```python
from build123d import *

# Parameters (mm, degrees)
PROFILE_R   = 4.7625
PROFILE_R_2 = 3.8735


with BuildPart() as part:
    # Tube: sweep along a curve in space
    with BuildLine() as tube_path:
        Line((-2198.887960479, -22.400788354, -83.600880265), (-2179.087960479, -22.400788354, -83.600880265))
        Line((-2179.087960479, -22.400788354, -83.600880265), (-2172.876303396, -22.612445436, -84.390795251))
        Line((-2172.876303396, -22.612445436, -84.390795251), (-2167.087960479, -23.232992603, -86.706708807))
        Line((-2167.087960479, -23.232992603, -86.706708807), (-2162.11739773, -24.220140591, -90.390795251))
        Line((-2162.11739773, -24.220140591, -90.390795251), (-2158.303350788, -25.506616895, -95.191990181))
        Line((-2158.303350788, -25.506616895, -95.191990181), (-2155.905740648, -27.004750281, -100.783100096))
        Line((-2155.905740648, -27.004750281, -100.783100096), (-2155.087960479, -28.612445436, -106.783100096))
        Line((-2155.087960479, -28.612445436, -106.783100096), (-2155.087960479, -33.219424439, -123.976579804))
    # Profile → Tube (sweep)
    with BuildSketch(Plane(origin=(-2198.887960479, 0, 0), x_dir=(0, 0, -1), z_dir=(1, 0, 0))):
        with Locations((83.600880265, -22.400788354)):
            Circle(PROFILE_R)
        with Locations((83.600880265, -22.400788354)):
            Circle(PROFILE_R_2, mode=Mode.SUBTRACT)
    sweep(path=tube_path.line, transition=Transition.RIGHT)


solid = part.part
```
Geometry: final body of the model. Coordinates: model frame, mm. A direction names the side the tool comes from. Round coordinates to 2 decimals unless told otherwise and drop trailing zeros. Write each loop counter-clockwise with the first axis right and the second up, starting at its lowest first coordinate (ties: lowest second). Pieces come first, ordered by that corner, then holes.
Item 1: Set-up query: faces 1 (the face through (-2188.691, -20.97, -88.143)), 2 (the face through (-2152.101, -25.944, -103.738)). Return all of +Z, -Z, +X, -X, +Y, -Y with unobstructed straight access to the full face (end or side cutting, diameter ignored); none if empty.
Item 2: Pin query (flat end, axial travel): P1, Ø4, axis at x = -2172, y = -21, coming from the -Z side; P2, Ø10, axis at x = -2187.5, y = -23, coming from the -Z side; P3, Ø6, axis at x = -2193.5, y = -28, coming from the +Z side; P4, Ø1, axis at y = -25.5, z = -119, coming from the -X side. Return the tip coordinate at first contact, or that it passes through.
Item 3: Mould query, pull axis Y, two halves, no side actions, for faces 3 (the face through (-2162.47, -21.3, -86.41)), 4 (the face through (-2161.73, -23.77, -84.75)), 5 (the face through (-2198.888, -18.5, -82.6)). Classes: +Y half, -Y half, draft (parallel to the pull), parting line (faces both ways), or undercut.
Item 4: Material intervals for L1, parallel to X at y = -27, z = -91.5; L2, parallel to Z at x = -2184, y = -20.25; L3, parallel to X at y = -25.25, z = -97, sorted ascending.
Item 5: Section query A-A (x = -2185). Return loops of the section in (y, z) (1 decimal), plus the area to 3 significant figures.
Completed:
1. face 1: -X
1. face 2: none
2. P1: stops at z = -90.43
2. P2: stops at z = -88.36
2. P3: stops at z = -79.61
2. P4: passes through
3. face 3: undercut
3. face 4: parting line
3. face 5: draft
4. L1: x = -2166.54 to -2164.78, -2156.91 to -2155.56
4. L2: z = -87.85 to -86.82, -80.38 to -79.35
4. L3: x = -2162.95 to -2161.81, -2153.49 to -2152.51
5. outline: circle Ø9.5 at (-22.4, -83.6); hole circle Ø7.7 at (-22.4, -83.6)
5. area: 24.1 mm2
